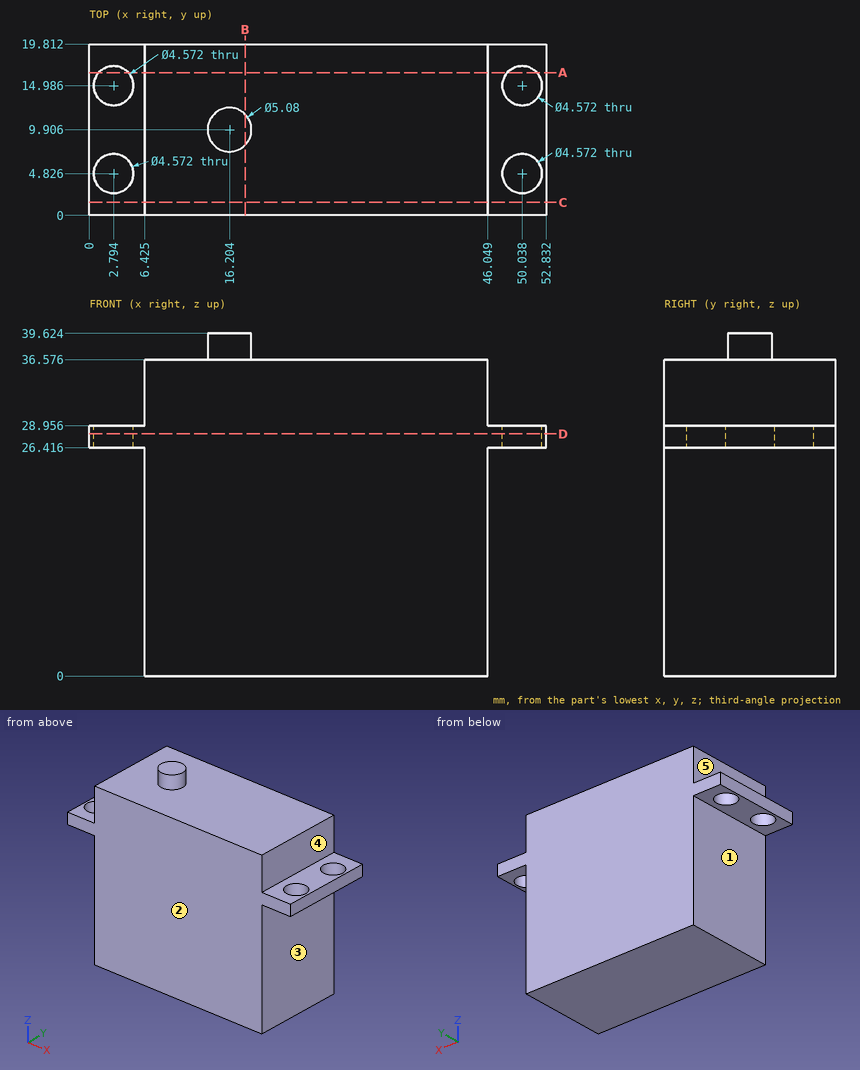
For this review, use the dimensioned drawing (mm, ordinates from the lowest corner) and the shaded views. A direction names the side the tool comes from. Round coordinates to 2 decimals unless told otherwise and drop trailing zeros. Loops run counter-clockwise (first coordinate to the right, second up) from the corner with the lowest first, then second, coordinate; pieces in that order, holes last. Notation, with made-up numbers: M 20,-39.75 L 50,-39.75 A15 ccw 50,-13.75 Z; hole C 10.25,89 d6. An arc over 180 degrees is marked long. Answer as CSV lines item,"result".
1. We need section C-C (y = 1.5). Give the boundary of the cut face in (x, z) (1 decimal).
Outcome:
outline,"M 0,26.4 L 6.4,26.4 L 6.4,0 L 46,0 L 46,26.4 L 52.8,26.4 L 52.8,29 L 46,29 L 46,36.6 L 6.4,36.6 L 6.4,29 L 0,29 Z"
2. Insertion check: pin 1 Ø4 at (x, y) = (2.794, 4.826) entering from +Z; pin 2 Ø7.5 at (x, y) = (50.5, 7.5) entering from -Z; pin 3 Ø4 at (x, y) = (37.5, 15) entering from +Z; pin 4 Ø3 at (x, y) = (41.5, 13.5) entering from -Z. Each pin has a flat end and moves straight along its axis. Give the tip position at first contact, or say it passes through.
Outcome:
pin 1,"passes through"
pin 2,"stops at z = 26.42"
pin 3,"stops at z = 36.58"
pin 4,"stops at z = 0"
3. For the marked faces 1, 2, 3, 4 and 5, list the 3-axis set-ups (+Z, -Z, +X, -X, +Y, -Y) from which the entire face can be reached by the end or side of a thin tool; tool diameter is ignored.
Outcome:
face 1,"-Z, -X, +Y, -Y"
face 2,"+Z, -Z, +X, -X, -Y"
face 3,"-Z, +X, +Y, -Y"
face 4,"+Z, +X, +Y, -Y"
face 5,"+Z, -X, +Y, -Y"
4. We need section D-D (z = 28). Give the boundary of the cut face in (x, y).
Outcome:
outline,"M 0,0 L 52.83,0 L 52.83,19.81 L 0,19.81 Z; hole C 2.79,4.83 d4.57; hole C 2.79,14.99 d4.57; hole C 50.04,4.83 d4.57; hole C 50.04,14.99 d4.57"
5. We need section B-B (x = 18). Give the boundary of the cut face in (y, z), plus the area to 3 significant figures.
Outcome:
outline,"M 0,0 L 19.81,0 L 19.81,36.58 L 11.7,36.58 L 11.7,39.62 L 8.11,39.62 L 8.11,36.58 L 0,36.58 Z"
area,"736 mm2"
6. To check wall thickness, follow L1, parallel to Z at x = 42, y = 5; L2, parallel to Z at x = 4, y = 7.5; L3, parallel to X at y = 6, z = 8.5 (1 decimal). State the ranges of each line that lie inside material, in increasing order. Write a range as [from, to].
Outcome:
L1,"z = [0, 36.58]"
L2,"z = [26.42, 28.96]"
L3,"x = [6.4, 46]"
7. We need section A-A (y = 16.5). Give the boundary of the cut face in (x, z) (1 decimal).
Outcome:
outline,"M 0,26.4 L 1.1,26.4 L 1.1,29 L 0,29 Z; M 4.5,26.4 L 6.4,26.4 L 6.4,0 L 46,0 L 46,26.4 L 48.3,26.4 L 48.3,29 L 46,29 L 46,36.6 L 6.4,36.6 L 6.4,29 L 4.5,29 Z; M 51.8,26.4 L 52.8,26.4 L 52.8,29 L 51.8,29 Z"
